Geometry check sheet. Reference: the model listing, model coordinates, mm. A direction names the side the tool comes from. Give positions to 0.01 mm unless a question says otherwise; leave off trailing zeros. Loops run counter-clockwise (first coordinate to the right, second up) from the corner with the lowest first, then second, coordinate; pieces in that order, holes last. Notation, with made-up numbers: (25.5, 71) -> (53.5, 71) arc R20 ccw to (53.5, 82) -> close; hole circle Ø3 at (-27, -17). An arc over 180 degrees is marked (long way). One line per item, written item: value. Start each with the question number.
(1) Sectioned sample at A-A, the plane y = -10. Record the cut outline in (x, z), then the cut area to 3 significant figures.
(2) Tool access check on faces 1 (the face through (-66.236, -11, 0)), 2 (the face through (23.764, -17, 0)), 3 (the face through (-29.396, -7.518, 0.151)). Record the directions out of +Z, -Z, +X, -X, +Y, -Y that give a thin tool (end or side, any length) a straight path to the whole face; none if there is none.
(3) Scan lines: line 1 along Y through (x, z) = (-7, 1); line 2 along Y through (x, z) = (-35, -2.5); line 3 along Z through (x, y) = (-56, -11.5). Record each from-to range of solid material in increasing order. Write a range as from..to.
(4) Sectioned sample at B-B, the plane x = -13. Record the cut outline in (y, z), then the cut area to 3 significant figures.
(5) Gauge pin test, flat ends, axial feed: pin 1 Ø1.1 at (y, z) = (-9.5, 1) entering from -X; pin 2 Ø2.5 at (y, z) = (-10, -1.5) entering from +X. Record the tip position at first contact, or that the pin passes through.
from build123d import *

# Parameters (mm, degrees)
BOSS_EXTRUDE1_DEPTH = 8
SKETCH2_W           = 135
SKETCH2_H           = 8.056190957
BOSS_EXTRUDE2_DEPTH = 10


with BuildPart() as part:
    # Sketch1 → Boss-Extrude1 (new body)
    with BuildSketch(Plane(origin=(0, 0, -3.792826984), x_dir=(-1, 0, 0), z_dir=(0, 0, -1))):
        Polygon((23.516961809, -6.40864854), (22.698028781, -8.65864854), (21.809158042, -8.65864854), (21.235890512, -7.083608945), (21.235890512, -12.40864854), (66.235890512, -12.40864854), (66.235890512, -8.65864854), (65.791455142, -8.65864854), (64.972522115, -6.40864854), (64.357666259, -6.40864854), (63.538733231, -8.65864854), (62.649862492, -8.65864854), (61.830929465, -6.40864854), (61.216073609, -6.40864854), (60.397140581, -8.65864854), (59.508269842, -8.65864854), (58.689336815, -6.40864854), (58.074480959, -6.40864854), (57.255547931, -8.65864854), (56.366677192, -8.65864854), (55.547744165, -6.40864854), (54.932888309, -6.40864854), (54.113955281, -8.65864854), (53.225084542, -8.65864854), (52.406151515, -6.40864854), (51.791295659, -6.40864854), (50.972362631, -8.65864854), (50.083491892, -8.65864854), (49.264558865, -6.40864854), (48.649703009, -6.40864854), (47.830769981, -8.65864854), (46.941899242, -8.65864854), (46.122966215, -6.40864854), (45.508110359, -6.40864854), (44.689177331, -8.65864854), (43.800306592, -8.65864854), (42.981373565, -6.40864854), (42.366517709, -6.40864854), (41.547584681, -8.65864854), (40.658713942, -8.65864854), (39.839780915, -6.40864854), (39.224925059, -6.40864854), (38.405992031, -8.65864854), (37.517121292, -8.65864854), (36.698188265, -6.40864854), (36.083332409, -6.40864854), (35.264399381, -8.65864854), (34.375528642, -8.65864854), (33.556595615, -6.40864854), (32.941739759, -6.40864854), (32.122806731, -8.65864854), (31.233935992, -8.65864854), (30.415002965, -6.40864854), (29.800147109, -6.40864854), (28.981214081, -8.65864854), (28.092343342, -8.65864854), (27.273410315, -6.40864854), (26.658554459, -6.40864854), (25.839621431, -8.65864854), (24.950750692, -8.65864854), (24.131817665, -6.40864854), align=None)
    extrude(amount=-BOSS_EXTRUDE1_DEPTH)

    # Sketch2 → Boss-Extrude2 (add)
    with BuildSketch(Plane.XZ.offset(12.40864854)):
        with Locations((-43.735890512, 0.179077538)):
            Rectangle(SKETCH2_W, SKETCH2_H)
    extrude(amount=BOSS_EXTRUDE2_DEPTH)


solid = part.part
Calculated:
1. outline: (-66.24, -3.79) -> (-21.24, -3.79) -> (-21.24, 4.21) -> (-66.24, 4.21) -> close
1. area: 360 mm2
2. face 1: +Z, -Z, -X, +Y
2. face 2: +Z, -Z, +X, +Y, -Y
2. face 3: +Z, -Z, +Y
3. line 1: y = -22.41..-12.41
3. line 2: y = -22.41..-8.66
3. line 3: z = -3.79..4.21
4. outline: (-22.41, -3.85) -> (-12.41, -3.85) -> (-12.41, 4.21) -> (-22.41, 4.21) -> close
4. area: 80.6 mm2
5. pin 1: stops at x = -66.24
5. pin 2: stops at x = -21.24
